The figure shows three views and two pictorial views of one solid part (mm, origin at its lowest corner). Answer the questions. A direction names the side the tool comes from. Round coordinates to 2 decimals unless told otherwise and drop trailing zeros. Order: outer loops, then holes, each group sorted by start corner. A loop starts at its lowest first (then second) coordinate and runs counter-clockwise, first axis right, second up. Notation, with made-up numbers: (-34, -6.75) - (-26, -6.75) arc R32 cw to (-26, 25.25) - close; hole circle Ø3 at (64, 45.5). An arc over 180 degrees is marked (long way). Answer as a JSON object with one key per item and string values. Group by question number.
Q1. A cutting plane is placed at A-A on y = 7.5. Determine the outline of the cut face in (x, z).
Q2. A cutting plane is placed at B-B on z = 97. Determine the outline of the cut face in (x, y).
Q3. The mould has two halves that part along Z. Classify the marked faces 3, 4 and 5: pulls with the +Z half, pulls with the -Z half, needs draft (parallel to the pull), parting line crosses it, or undercut.
Q4. Consider line 1 (Z direction, x = 34.5, y = 71.5) (1 decimal); line 2 (X direction, y = 48.5, z = 135.5); line 3 (Z direction, x = 57, y = 10.5). Determine where each line is inside the solid, lowest interval first.
Q5. A cutting plane is placed at D-D on y = 45.5. Determine the outline of the cut face in (x, z) (1 decimal).
Q6. A tool of negligible diameter and unlimited length cuts with its end or side. For the marked faces 1 and 2, from which of +Z, -Z, +X, -X, +Y, -Y can it reach the whole face along a straight path? Write none if from no direction.
Q7. A cutting plane is placed at C-C on x = 73. Determine the outline of the cut face in (y, z) (1 decimal).
Q8. Given pin 1 Ø8 at (y, z) = (55.5, 91.5) entering from -X; pin 2 Ø6 at (x, z) = (122.5, 18.5) entering from -Y; pin 3 Ø1 at (x, z) = (44.5, 56) entering from -Y, each flat-ended and moving along its own axis, determine where each tip first touches the part or whether it passes through.
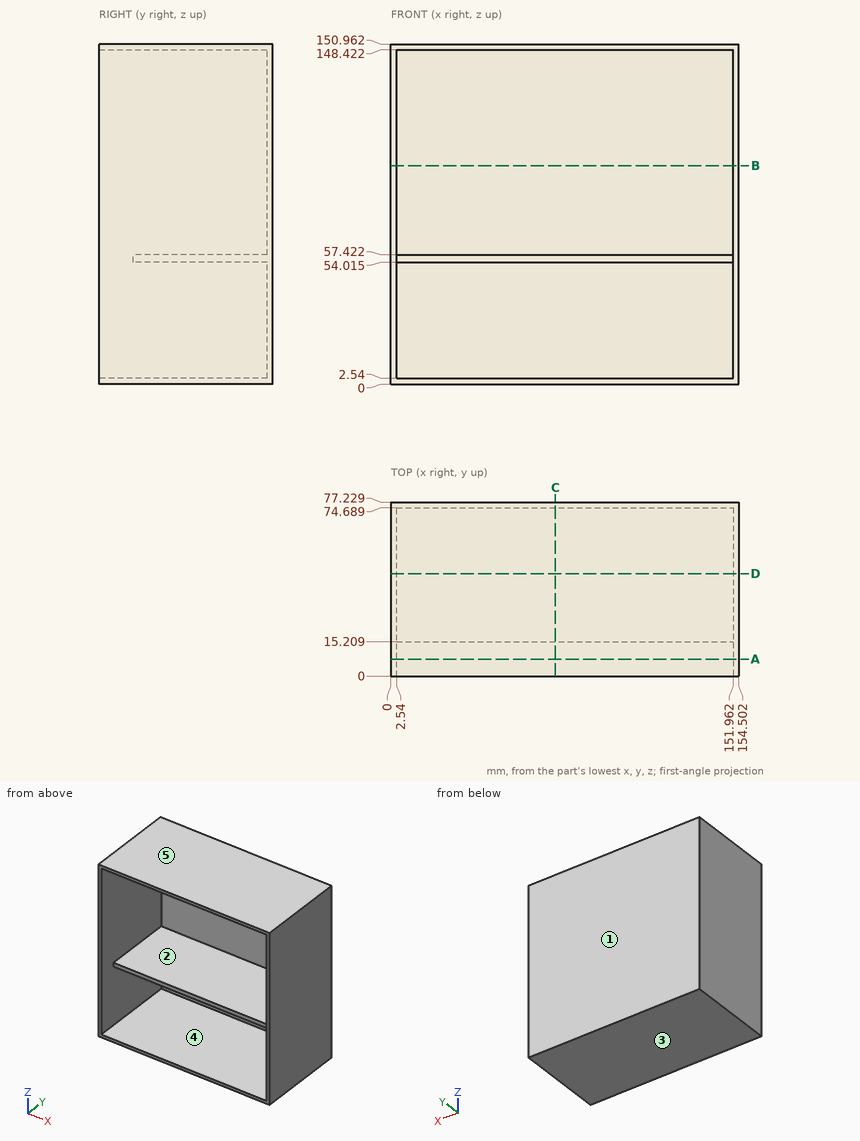
Result set:
{
 "1": {"outline": "(0, 0) - (154.5, 0) - (154.5, 150.96) - (0, 150.96) - close; hole (2.54, 2.54) - (151.96, 2.54) - (151.96, 148.42) - (2.54, 148.42) - close"},
 "2": {"outline": "(0, 0) - (2.54, 0) - (2.54, 74.69) - (151.96, 74.69) - (151.96, 0) - (154.5, 0) - (154.5, 77.23) - (0, 77.23) - close"},
 "3": {"face 3": "pulls with the -Z half", "face 4": "undercut", "face 5": "pulls with the +Z half"},
 "4": {"line 1": "z = 0 to 2.5, 54 to 57.4, 148.4 to 151", "line 2": "x = 0 to 2.54, 151.96 to 154.5", "line 3": "z = 0 to 2.54, 148.42 to 150.96"},
 "5": {"outline": "(0, 0) - (154.5, 0) - (154.5, 151) - (0, 151) - close; hole (2.5, 2.5) - (152, 2.5) - (152, 54) - (2.5, 54) - close; hole (2.5, 57.4) - (152, 57.4) - (152, 148.4) - (2.5, 148.4) - close"},
 "6": {"face 1": "+Z, -Z, +X, -X, +Y", "face 2": "-Y"},
 "7": {"outline": "(0, 0) - (77.2, 0) - (77.2, 151) - (0, 151) - (0, 148.4) - (74.7, 148.4) - (74.7, 57.4) - (15.2, 57.4) - (15.2, 54) - (74.7, 54) - (74.7, 2.5) - (0, 2.5) - close"},
 "8": {"pin 1": "stops at x = 0", "pin 2": "stops at y = 74.69", "pin 3": "stops at y = 15.21"}
}
